Here's how the part is built. I have some questions about the finished solid (model axes, mm). Face numbers are marked on the shaded views. A direction names the side the tool comes from. Give positions to 0.01 mm unless a question says otherwise; leave off trailing zeros. Write each loop counter-clockwise with the first axis right and the second up, starting at its lowest first coordinate (ties: lowest second). Pieces come first, ordered by that corner, then holes. Notation, with made-up numbers: M -22.75,-5.5 L 35.25,-5.5 A21 ccw 35.25,20.5 Z; hole C 29,-2.5 d2. An arc over 180 degrees is marked long. Answer as CSV lines item,"result". Start each with the question number.
Q1. Suppose I cut it at C-C (y = -6). Count the separate pieces of the cut face and the enclosed holes in it, then the cut area to 3 significant figures.
Q2. Suppose I cut it at A-A (y = -11). Write out the boundary of the cut face in (x, z).
Q3. Suppose I cut it at B-B (x = 17.5). Write out the boundary of the cut face in (y, z).
Q4. On a 3-axis mill with a long thin cutter (end or side, diameter ignored), from which of +Z, -Z, +X, -X, +Y, -Y can I reach the whole of each face in a straight line? I mean the marked faces 4 and 5. Say none if no direction works.
Q5. If I drill on line 1 along Y through (x, z) = (31.75, 4); line 2 along X through (y, z) = (-2.5, 2.75); line 3 along Y through (x, z) = (34, 2.5), over which ranges is the centre line in solid material (lowest first)?
Q6. Thinking about a two-plate mould opening in X: for the marked faces 1, 2 and 3, which applies, +X half, -X half, draft (parallel to the pull), parting line (faces both ways), or undercut?
Q7. For pin 1 (2.5 mm diameter, centred on x = 17.5, z = 5.5, fed in from -Y); pin 2 (4 mm diameter, centred on y = -12, z = 1.5, fed in from -X), each with a flat end and sliding along its axis, tell me the tip position at first contact or that it passes through.
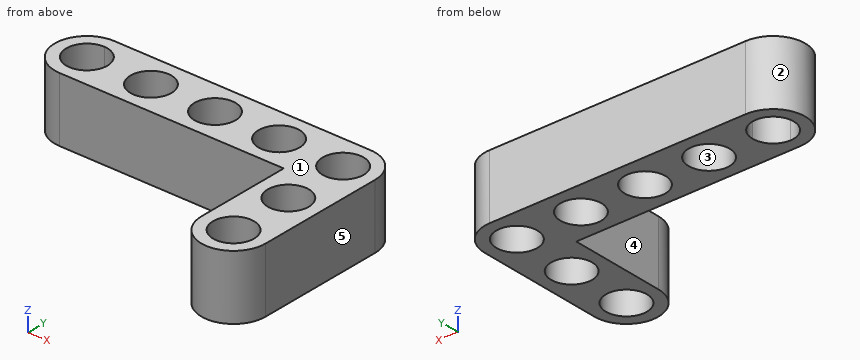
```python
from build123d import *

# Parameters (mm, degrees)
F0_R     = 2.54
F1_DEPTH = 7.9375


with BuildPart() as f1:
    # F0 (on Top) → F1 (new body)
    with BuildSketch(Plane.XY):
        with BuildLine():
            Line((31.75, 0), (0, 0))
            Line((0, 0), (0, -1.42875))
            ThreePointArc((0, -1.42875), (1.796051, -2.172699), (2.54, -3.96875))
            ThreePointArc((2.54, -3.96875), (1.796051, -5.764801), (0, -6.50875))
            Line((0, -6.50875), (0, -7.9375))
            Line((0, -7.9375), (27.78125, -7.9375))
            Line((27.78125, -7.9375), (27.78125, -19.84375))
            ThreePointArc((27.78125, -19.84375), (31.75, -23.8125), (35.71875, -19.84375))
            Line((35.71875, -19.84375), (35.71875, -3.96875))
            ThreePointArc((35.71875, -3.96875), (34.55633, -1.16242), (31.75, 0))
        make_face()
        with Locations((31.75, -19.84375)):
            Circle(F0_R, mode=Mode.SUBTRACT)
        with Locations((7.9375, -3.96875)):
            Circle(F0_R, mode=Mode.SUBTRACT)
        with Locations((31.75, -11.90625)):
            Circle(F0_R, mode=Mode.SUBTRACT)
        with Locations((15.875, -3.96875)):
            Circle(F0_R, mode=Mode.SUBTRACT)
        with Locations((23.8125, -3.96875)):
            Circle(F0_R, mode=Mode.SUBTRACT)
        with Locations((31.75, -3.96875)):
            Circle(F0_R, mode=Mode.SUBTRACT)
        with BuildLine():
            Line((0, -1.42875), (0, 0))
            ThreePointArc((0, 0), (-3.96875, -3.96875), (0, -7.9375))
            Line((0, -7.9375), (0, -6.50875))
            ThreePointArc((0, -6.50875), (-2.54, -3.96875), (0, -1.42875))
        make_face()
    extrude(amount=F1_DEPTH)


solid = f1.part
```
Resolved:
1,separate pieces,"6"
1,enclosed holes,"0"
1,area,"190 mm^2"
2,outline,"M 27.78,0 L 29.38,0 L 29.38,7.94 L 27.78,7.94 Z; M 34.12,0 L 35.72,0 L 35.72,7.94 L 34.12,7.94 Z"
3,outline,"M -7.94,0 L -5.92,0 L -5.92,7.94 L -7.94,7.94 Z; M -2.02,0 L 0,0 L 0,7.94 L -2.02,7.94 Z"
4,face 4,"+Z, -Z, -X, -Y"
4,face 5,"+Z, -Z, +X, +Y, -Y"
5,line 1,"-23.81 to -22.38, -17.3 to -14.45, -9.37 to -6.51, -1.43 to 0"
5,line 2,"-3.69 to -2.07, 2.07 to 5.87, 10.01 to 13.8, 17.95 to 21.74, 25.88 to 29.68, 33.82 to 35.44"
5,line 3,"-23.11 to -21.02, -18.67 to -13.08, -10.73 to -5.15, -2.79 to -0.7"
6,face 1,"draft"
6,face 2,"-X half"
6,face 3,"undercut"
7,pin 1,"y = -7.94"
7,pin 2,"x = 27.78"
